```python
from build123d import *

# Parameters (mm, degrees)
F0_R           = 33.3375
F1_DEPTH       = 50.8
F2_T           = -1.5875
F6_W           = 2.5429241359
F6_H           = 13.1887868047
F7_DEPTH       = 12.7
F10_W          = 2.6744855568
F10_H          = 12.775093317
F11_DEPTH      = 2.794
F11_DEPTH_BACK = 2.413
F13_W          = 2.5820170995
F13_H          = 12.7615630627
F14_DEPTH      = 5.0546
F14_DEPTH_BACK = 4.7244
F15_W          = 7.62
F15_H          = 31.75
F15_R          = 1.397
F16_DEPTH      = 9.906


# Not quite as in the source:
# - a feature names something its author has since deleted; it is built from what else it names


with BuildPart() as f1:
    # F0 (on Top) → F1 (new body)
    with BuildSketch(Plane.XY):
        Circle(F0_R)
    extrude(amount=F1_DEPTH)

    # F2
    f2_openings = [f1.faces().sort_by_distance(p)[0] for p in [
        (0, 0, 50.8),
    ]]
    offset(amount=F2_T, openings=f2_openings)

    # F6 (on offset) → F7 (cut)
    with BuildSketch(Plane(origin=(-28.8711218987, -16.66875, 0), x_dir=(0.5, -0.8660254038, 0), z_dir=(-0.8660254038, -0.5, 0))):
        with Locations((0, 44.4019660354)):
            Rectangle(F6_W, F6_H)
    extrude(amount=-F7_DEPTH, mode=Mode.SUBTRACT)

    # F10 (on offset) → F11 (cut, two sides)
    with BuildSketch(Plane(origin=(28.8161292855, -16.637, 0), x_dir=(0.5, 0.8660254038, 0), z_dir=(0.8660254038, -0.5, 0))) as f11_sk:
        with Locations((0, 44.3391613662)):
            Rectangle(F10_W, F10_H)
    extrude(amount=-F11_DEPTH, mode=Mode.SUBTRACT)
    extrude(f11_sk.sketch, amount=F11_DEPTH_BACK, mode=Mode.SUBTRACT)

    # F13 (on offset) → F14 (cut, two sides)
    with BuildSketch(Plane.XZ.offset(-33.81375)) as f14_sk:
        with Locations((0, 44.5175170898)):
            Rectangle(F13_W, F13_H)
    extrude(amount=-F14_DEPTH, mode=Mode.SUBTRACT)
    extrude(f14_sk.sketch, amount=F14_DEPTH_BACK, mode=Mode.SUBTRACT)

    # F15 (on Top) → F16 (cut)
    with BuildSketch(Plane.XY):
        with Locations((-8.89, 0)):
            Rectangle(F15_W, F15_H)
        with Locations((-21.6036192909, 4.2545016563)):
            Circle(F15_R)
        with Locations((3.7963807091, 4.2545016563)):
            Circle(F15_R)
        with Locations((-8.9036192909, 22.3520016563)):
            Circle(F15_R)
    extrude(amount=F16_DEPTH, mode=Mode.SUBTRACT)


solid = f1.part
```
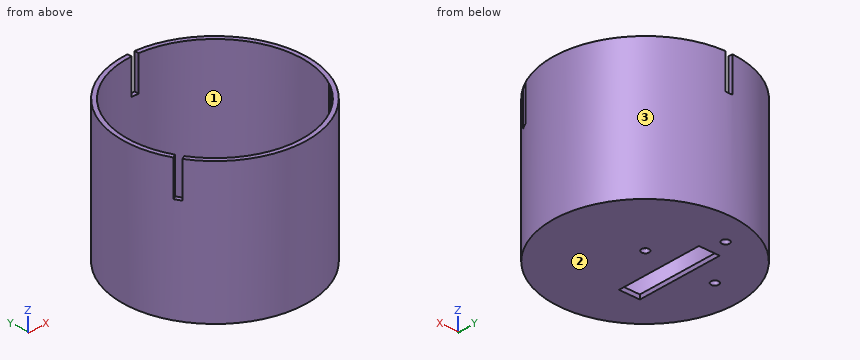
Source: CAD feature listing. Evaluate the final solid. Frame: model axes, mm. Face numbers are marked on the shaded views. Give positions to 0.01 mm unless a question says otherwise; leave off trailing zeros. Write each loop counter-clockwise with the first axis right and the second up, starting at its lowest first coordinate (ties: lowest second). Pieces come first, ordered by that corner, then holes. Notation, with made-up numbers: (64.25, 26) - (112.25, 26) arc R28 cw to (112.25, 45) - close; hole circle Ø9 at (54.5, 71). An arc over 180 degrees is marked (long way). One line per item, written item: value. Start each with the question number.
Q1. Material intervals for probe 1 along X at (y, z) = (0, 39); probe 2 along Y at (x, z) = (0, 40), sorted ascending. Write a range as from..to.
Q2. Draft query along Y for the marked faces 1, 2 and 3. Return one class per face: +Y half, -Y half, draft (parallel to the pull), parting line (faces both ways), or undercut.
Q3. First-contact query: pin 1 Ø3 at (x, y) = (3.8, 4.25) entering from +Z; pin 2 Ø0.5 at (y, z) = (-1.5, 0.5) entering from -X; pin 3 Ø1.7 at (x, z) = (-7, 0.5) entering from -Y. Flat tips, straight axial feed; report the tip coordinate or a pass-through.
Q4. Section query D-D, the plane y = -23. Return the cut outline in (x, z), then the cut area to 3 significant figures.
Q5. Section query B-B, the plane y = 0. Return the cut outline in (x, z).
Q6. Section query C-C, the plane x = 0. Return the cut outline in (y, z).
Q7. Section query A-A, the plane z = 45. Count the separate pieces of the cut face and the enclosed holes in it, then the cut area to 3 significant figures.
Answer:
1. probe 1: x = -33.34..-31.75, 31.75..33.34
1. probe 2: y = -33.34..-31.75
2. face 1: undercut
2. face 2: draft
2. face 3: parting line
3. pin 1: stops at z = 1.59
3. pin 2: stops at x = -33.31
3. pin 3: stops at y = -32.77
4. outline: (-24.13, 0) - (24.13, 0) - (24.13, 50.8) - (21.89, 50.8) - (21.89, 1.59) - (-21.89, 1.59) - (-21.89, 50.8) - (-24.13, 50.8) - close
4. area: 298 mm2
5. outline: (-33.34, 0) - (-12.7, 0) - (-12.7, 1.59) - (-31.75, 1.59) - (-31.75, 50.8) - (-33.34, 50.8) - close; (-5.08, 0) - (33.34, 0) - (33.34, 50.8) - (31.75, 50.8) - (31.75, 1.59) - (-5.08, 1.59) - close
6. outline: (-33.34, 0) - (33.34, 0) - (33.34, 38.14) - (31.75, 38.14) - (31.75, 1.59) - (-31.75, 1.59) - (-31.75, 50.8) - (-33.34, 50.8) - close
7. separate pieces: 3
7. enclosed holes: 0
7. area: 312 mm2
